```python
from build123d import *

# Parameters (mm, degrees)
SKETCH1_R           = 1.5
SKETCH1_W           = 5
SKETCH1_H           = 5
BOSS_EXTRUDE1_DEPTH = 5
FILLET3_R           = 1


with BuildPart() as part:
    # Sketch1 → Boss-Extrude1 (new body)
    with BuildSketch(Plane.XY):
        Polygon((0, 5), (0, 19.982808697), (0, 31), (0, 30.1), (0, 47), (10.2, 47), (10.2, 44), (8.2, 44), (8.2, 42.4), (12.2, 42.4), (12.2, 38.3), (8.2, 38.3), (8.2, 36.7), (22.2, 36.7), (22.2, 32.6), (18.2, 32.6), (18.2, 31), (32.2, 31), (32.2, 26.9), (28.2, 26.9), (28.2, 25.3), (42.2, 25.3), (42.2, 21.2), (38.2, 21.2), (38.2, 19.6), (58.2, 19.6), (58.2, 5), (20, 5), (20, 0), (15, 0), (15, 5), (11.5, 5), (11.5, 8), (12.6, 8), (12.6, 10.3), (11.5, 10.3), (11.5, 15), (8.5, 15), (8.5, 10.3), (7.4, 10.3), (7.4, 8), (8.5, 8), (8.5, 5), (5, 5), (5, 0), (0, 0), align=None)
        with Locations((45.7, 15.15)):
            Circle(SKETCH1_R, mode=Mode.SUBTRACT)
        with Locations((40.7, 15.15)):
            Rectangle(SKETCH1_W, SKETCH1_H, mode=Mode.SUBTRACT)
        with Locations((50.7, 15.15)):
            Rectangle(SKETCH1_W, SKETCH1_H, mode=Mode.SUBTRACT)
    extrude(amount=BOSS_EXTRUDE1_DEPTH)

    # Fillet3
    fillet3_edges = [part.edges().sort_by_distance(p)[0] for p in [
        (10.2, 44, 2.5),
        (12.2, 42.4, 2.5),
        (12.2, 38.3, 2.5),
        (22.2, 36.7, 2.5),
        (22.2, 32.6, 2.5),
        (32.2, 31, 2.5),
        (32.2, 26.9, 2.5),
        (42.2, 25.3, 2.5),
        (42.2, 21.2, 2.5),
    ]]
    fillet(fillet3_edges, radius=FILLET3_R)


solid = part.part
```
Geometry check sheet. Reference: the model listing, model coordinates, mm. A direction names the side the tool comes from. Round coordinates to 2 decimals unless told otherwise and drop trailing zeros. Order: outer loops, then holes, each group sorted by start corner. A loop starts at its lowest first (then second) coordinate and runs counter-clockwise, first axis right, second up. Notation, with made-up numbers: (7, 40.25) - (30, 40.25) arc R9 cw to (30, 45.25) - close; hole circle Ø2 at (47.5, -18.75). An arc over 180 degrees is marked (long way). Use a Markdown table: item, result. Add a question column.
(1) Tool access check on faces 4 (the flat face through (12.2, 40, 2)), 5 (the flat face through (38.2, 20, 2)), 6 (the flat face through (20, 3, 2)), 7 (the flat face through (7, 5, 2)). Record the directions out of +Z, -Z, +X, -X, +Y, -Y that give a thin tool (end or side, any length) a straight path to the whole face; none if there is none.
(2) Sectioned sample at A-A, the plane x = 45.7. Enter the section's corners in (y, z).
(3) Depth check by flat-ended pin: pin 1 (0.8 mm diameter, centred on y = 32, z = 2.5, fed in from +X); pin 2 (1.8 mm diameter, centred on y = 38, z = 2, fed in from +X); pin 3 (1 mm diameter, centred on y = 46, z = 2.5, fed in from +X). Enter the tip coordinate at first touch or a pass-through.
(4) Sectioned sample at C-C, the plane y = 29. Enter the section's corners in (x, z).
(5) Sectioned sample at B-B, the plane y = 6.5. Enter the section's corners in (x, z), and give its area (3 significant figures).
(6) Sectioned sample at D-D, the plane z = 1.55. Count the separate pieces of the cut face and the enclosed holes in it, and give its area (3 significant figures).
(7) Release check for a two-part mould opening along Y. For faces 1 (the flat face through (10, 15, 2)), 2 (the flat face through (8.2, 38, 2)), 3 (the flat face through (11.5, 6, 2)) record: pulls with the +Y half, pulls with the -Y half, needs draft (parallel to the pull), parting line crosses it, or undercut.
(8) Material ranges on line 1 along Y through (x, z) = (48.5, 4.55); line 2 along Y through (x, z) = (21, 0.45); line 3 along X through (y, z) = (41.5, 3.25), recorded low to high. Write a range as [from, to].
Answers below:
| question | item | result |
|---|---|---|
| 1 | face 4 | +Z, -Z, +X, +Y |
| 1 | face 5 | +Z, -Z, +X |
| 1 | face 6 | +Z, -Z, +X, -Y |
| 1 | face 7 | +Z, -Z, -Y |
| 2 | outline | (5, 0) - (13.65, 0) - (13.65, 5) - (5, 5) - close; (16.65, 0) - (19.6, 0) - (19.6, 5) - (16.65, 5) - close |
| 3 | pin 1 | x = 18.2 |
| 3 | pin 2 | x = 12.12 |
| 3 | pin 3 | x = 10.2 |
| 4 | outline | (0, 0) - (32.2, 0) - (32.2, 5) - (0, 5) - close |
| 5 | outline | (0, 0) - (8.5, 0) - (8.5, 5) - (0, 5) - close; (11.5, 0) - (58.2, 0) - (58.2, 5) - (11.5, 5) - close |
| 5 | area | 276 mm² |
| 6 | separate pieces | 1 |
| 6 | enclosed holes | 3 |
| 6 | area | 1,440 mm² |
| 7 | face 1 | pulls with the -Y half |
| 7 | face 2 | undercut |
| 7 | face 3 | needs draft |
| 8 | line 1 | [5, 12.65], [17.65, 19.6] |
| 8 | line 2 | [5, 31], [32.6, 36.7] |
| 8 | line 3 | [0, 12.19] |
